```python
from build123d import *

# Parameters (mm, degrees)
ESQUISSE1_W        = 8
ESQUISSE1_H        = 10
BOSS_EXTRU_1_DEPTH = 4
ESQUISSE2_W        = 0.201235696
ESQUISSE2_H        = 0.359902984
BOSS_EXTRU_2_DEPTH = 4
ESQUISSE3_R        = 2.6
BOSS_EXTRU_3_DEPTH = 3
ESQUISSE4_R        = 0.5
BOSS_EXTRU_4_DEPTH = 9


with BuildPart() as part:
    # Esquisse1 → Boss.-Extru.1 (new body)
    with BuildSketch(Plane(origin=(0, 0, 0), x_dir=(0, 0, -1), z_dir=(1, 0, 0))):
        Rectangle(ESQUISSE1_W, ESQUISSE1_H)
    extrude(amount=BOSS_EXTRU_1_DEPTH)

    # Esquisse2 → Boss.-Extru.2 (add)
    with BuildSketch(Plane.XZ.offset(5)):
        with Locations((2, 2.580715462)):
            Rectangle(ESQUISSE2_W, ESQUISSE2_H)
    boss_extru_2 = extrude(amount=BOSS_EXTRU_2_DEPTH)

    # Symétrie1: Boss.-Extru.2 across plane
    add(boss_extru_2.mirror(Plane.XY))

    # Esquisse3 → Boss.-Extru.3 (add)
    with BuildSketch(Plane(origin=(0, 5, 0), x_dir=(1, 0, 0), z_dir=(0, 1, 0))):
        with Locations(Location((2, 0, 0), (0, 0, 39.715137232))):
            Circle(ESQUISSE3_R)
    extrude(amount=BOSS_EXTRU_3_DEPTH)

    # Esquisse4 → Boss.-Extru.4 (add)
    with BuildSketch(Plane(origin=(0, 8, 0), x_dir=(1, 0, 0), z_dir=(0, 1, 0))):
        with Locations(Location((2.053541677, 0, 0), (0, 0, 270))):
            Circle(ESQUISSE4_R)
    extrude(amount=BOSS_EXTRU_4_DEPTH)


solid = part.part
```
Geometry: final body of the model. Coordinates: model frame, mm. A direction names the side the tool comes from. Round coordinates to 2 decimals unless told otherwise and drop trailing zeros. Loops run counter-clockwise (first coordinate to the right, second up) from the corner with the lowest first, then second, coordinate; pieces in that order, holes last. Notation, with made-up numbers: (-26.75, 55) -> (26.25, 55) arc R12 ccw to (26.25, 73) -> close; hole circle Ø8 at (49, 63.5). An arc over 180 degrees is marked (long way). Write each question's results on one line, items separated by ' | '.
Item 1: Cut plane D-D on y = 15. Return the cut outline in (x, z), and give its area (3 significant figures).
Answers below:
outline: circle Ø1 at (2.05, 0) | area: 0.785 mm²
Item 2: Cut plane B-B on y = -0.25. Return the cut outline in (x, z).
Answers below:
outline: (0, -4) -> (4, -4) -> (4, 4) -> (0, 4) -> close
Item 3: Cut plane C-C on z = -2. Return the cut outline in (x, y), and give its area (3 significant figures).
Answers below:
outline: (0, -5) -> (4, -5) -> (4, 5) -> (3.66, 5) -> (3.66, 8) -> (0.34, 8) -> (0.34, 5) -> (0, 5) -> close | area: 50.0 mm²
Item 4: Set-up query: faces 1 (the face through (2, 0, -4)), 2 (the face through (4.4, 6.5, 1)), 3 (the face through (4, 0, 0)), 4 (the face through (0, 0, 0)). Return all of +Z, -Z, +X, -X, +Y, -Y with unobstructed straight access to the full face (end or side cutting, diameter ignored); none if empty.
Answers below:
face 1: -Z, +X, -X, +Y, -Y | face 2: +Y | face 3: +Z, -Z, +X, -Y | face 4: +Z, -Z, -X, -Y
Item 5: Pin query (flat end, axial travel): pin 1 Ø0.7 at (x, z) = (1, 3) entering from +Y; pin 2 Ø1.2 at (x, z) = (1.5, -1.5) entering from -Y; pin 3 Ø1 at (y, z) = (0, -2.5) entering from -X. Return the tip coordinate at first contact, or that it passes through.
Answers below:
pin 1: stops at y = 5 | pin 2: stops at y = -5 | pin 3: stops at x = 0
Item 6: Line query: probe 1 along Y at (x, z) = (1.35, -2.25); probe 2 along X at (y, z) = (3, 1.75); probe 3 along Y at (x, z) = (1.7, 0). Output: solid intervals per line, ascending. Write a range as [from, to].
Answers below:
probe 1: y = [-5, 8] | probe 2: x = [0, 4] | probe 3: y = [-5, 17]
Item 7: Cut plane A-A on z = 0. Return the cut outline in (x, y).
Answers below:
outline: (-0.6, 5) -> (0, 5) -> (0, -5) -> (4, -5) -> (4, 5) -> (4.6, 5) -> (4.6, 8) -> (2.55, 8) -> (2.55, 17) -> (1.55, 17) -> (1.55, 8) -> (-0.6, 8) -> close
